Part model, mm, in its own coordinate system. A direction names the side the tool comes from. Give positions to 0.01 mm unless a question says otherwise; leave off trailing zeros. Write each loop counter-clockwise with the first axis right and the second up, starting at its lowest first coordinate (ties: lowest second). Pieces come first, ordered by that corner, then holes.
Autodesk Inventor part; units mm, degrees
ref_plane "YZ Plane" through (0, 0, 0) normal (1, 0, 0) x (0, 1, 0)
ref_plane "XZ Plane" through (0, 0, 0) normal (0, 1, 0) x (-1, 0, 0)
ref_plane "XY Plane" through (0, 0, 0) normal (0, 0, 1) x (1, 0, 0)
sketch "Sketch1" plane through (0, 0, 0) normal (0, 0, 1) x (1, 0, 0)
  line L0 (0, 0) -> (65.7, 0)
  line L1 (65.7, 0) -> (65.7, 40.8)
  line L2 (0, 40.8) -> (0, 0)
  line L3 (0, 40.8) -> (-8, 40.8)
  line L4 (-8, 40.8) -> (-8, 44.8)
  line L5 (-8, 44.8) -> (0, 44.8)
  line L6 (0, 44.8) -> (4.8644, 57.5)
  line L7 (4.8644, 57.5) -> (49.9378, 57.5)
  line L8 (49.9378, 57.5) -> (64.8064, 44.8)
  line L9 (64.8064, 44.8) -> (72.8064, 44.8)
  line L10 (72.8064, 44.8) -> (72.8064, 40.8)
  line L11 (72.8064, 40.8) -> (65.7, 40.8)
  dimension "d0" = 65.7
  dimension "d1" = 40.8
  dimension "d2" = 4
  dimension "d9" = 57.5
  dimension "d13" = 8
  dimension "d14" = 8
extrude "Extrusion1" add sketch "Sketch1" against normal blind 30
sketch "Sketch2" plane through (4.8644, 57.5, 0) normal (0, 1, 0) x (1, 0, 0)
  circle A0 centre (10.1356, 15) radius 3.5
  line L0 (-12.8644, 30) -> (-4.8644, 30)
  point P0 (-4.8644, 0)
  dimension "d5" = 7
  dimension "d6" = 15
  dimension "d7" = 15
extrude "Extrusion2" add sketch "Sketch2" along normal blind 6.8
properties part number "servo60"
1) Drill centre lines: L1, parallel to Y at x = 24.5, z = -8.75; L2, parallel to X at y = 31, z = -22.75; L3, parallel to Y at x = 68, z = -16. Where is each one in solid material? Low to high.
Check result:
L1: y = 0 to 57.5
L2: x = 0 to 65.7
L3: y = 40.8 to 44.8
2) Flat gauge pins, fed straight in: P1, Ø4, axis at x = 70.5, z = -10, coming from the +Y side; P2, Ø3, axis at x = 43, z = -8, coming from the -Y side; P3, Ø2, axis at x = 9, z = -18, coming from the +Y side; P4, Ø15, axis at y = 17.5, z = -14.5, coming from the +X side. Where does each tip first touch, or does it go through?
Check result:
P1: stops at y = 44.8
P2: stops at y = 0
P3: stops at y = 57.5
P4: stops at x = 65.7
3) Saw through at D-D (x = -1). Write the cut outline in (y, z).
Check result:
outline: (40.8, -30) - (44.8, -30) - (44.8, 0) - (40.8, 0) - close
4) Saw through at B-B (z = -15). Write the cut outline in (x, y), and give its area (3 significant figures).
Check result:
outline: (-8, 40.8) - (0, 40.8) - (0, 0) - (65.7, 0) - (65.7, 40.8) - (72.81, 40.8) - (72.81, 44.8) - (64.81, 44.8) - (49.94, 57.5) - (18.5, 57.5) - (18.5, 64.3) - (11.5, 64.3) - (11.5, 57.5) - (4.86, 57.5) - (0, 44.8) - (-8, 44.8) - close
area: 3,750 mm2
5) Saw through at C-C (y = 11.5). Write the cut outline in (x, z), and give its area (3 significant figures).
Check result:
outline: (0, -30) - (65.7, -30) - (65.7, 0) - (0, 0) - close
area: 1,970 mm2
6) 3-axis set-ups, long thin cutter, end or side, ignore diameter. For faces 1 (the cylindrical face through (18.233, 60.852, -16.341)), 2 (the flat face through (-4, 40.8, -15)), 3 (the flat face through (65.7, 20, -15)): which of +Z, -Z, +X, -X, +Y, -Y reach the whole face in a straight line?
Check result:
face 1: +Y
face 2: +Z, -Z, -X, -Y
face 3: +Z, -Z, +X, -Y
7) Saw through at A-A (x = 15). Write the cut outline in (y, z).
Check result:
outline: (0, -30) - (57.5, -30) - (57.5, -18.5) - (64.3, -18.5) - (64.3, -11.5) - (57.5, -11.5) - (57.5, 0) - (0, 0) - close
